from build123d import *

# Parameters (mm, degrees)
SKETCH1_W           = 104.5
SKETCH1_H           = 70
BOSS_EXTRUDE1_DEPTH = 70
SKETCH2_W           = 94.7
SKETCH2_H           = 60.2
CUT_EXTRUDE1_DEPTH  = 11
CUT_EXTRUDE3_DEPTH  = 55
SKETCH5_W           = 20
SKETCH5_H           = 10
CUT_EXTRUDE4_DEPTH  = 10


with BuildPart() as part:
    # Sketch1 → Boss-Extrude1 (new body)
    with BuildSketch(Plane(origin=(0, 0, 0), x_dir=(1, 0, 0), z_dir=(0, 1, 0))):
        with Locations((52.25, 35)):
            Rectangle(SKETCH1_W, SKETCH1_H)
    extrude(amount=BOSS_EXTRUDE1_DEPTH)

    # Sketch2 → Cut-Extrude1 (cut)
    with BuildSketch(Plane(origin=(0, 70, 0), x_dir=(1, 0, 0), z_dir=(0, 1, 0))):
        with Locations((52.2, 35)):
            Rectangle(SKETCH2_W, SKETCH2_H)
    extrude(amount=-CUT_EXTRUDE1_DEPTH, mode=Mode.SUBTRACT)

    # Sketch3 → Cut-Extrude3 (cut)
    with BuildSketch(Plane(origin=(0, 59, 0), x_dir=(1, 0, 0), z_dir=(0, 1, 0))):
        with BuildLine():
            Line((99.5, 39.153311931), (99.5, 58))
            Line((99.5, 58), (90.5, 58))
            Line((90.5, 58), (90.5, 65))
            Line((90.5, 65), (60, 65))
            Line((60, 65), (60, 58))
            Line((60, 58), (13, 58))
            Line((13, 58), (13, 65))
            Line((13, 65), (5, 65))
            Line((5, 65), (5, 57))
            Line((5, 57), (12, 57))
            Line((12, 57), (12, 12))
            Line((12, 12), (30.952452159, 12))
            ThreePointArc((30.952452159, 12), (33.5, 6.1), (36.047547841, 12))
            Line((36.047547841, 12), (65.092654993, 12))
            ThreePointArc((65.092654993, 12), (68.5, 7.7), (71.907345007, 12))
            Line((71.907345007, 12), (76.805924131, 12))
            ThreePointArc((76.805924131, 12), (82.5, 5.45), (88.194075869, 12))
            Line((88.194075869, 12), (99.5, 12))
            Line((99.5, 12), (99.5, 30.846688069))
            ThreePointArc((99.5, 30.846688069), (100, 35), (99.5, 39.153311931))
        make_face()
    extrude(amount=-CUT_EXTRUDE3_DEPTH, mode=Mode.SUBTRACT)

    # Sketch5 → Cut-Extrude4 (cut)
    with BuildSketch(Plane(origin=(104.5, 0, 0), x_dir=(0, 0, -1), z_dir=(1, 0, 0))):
        with Locations((35, 10)):
            Rectangle(SKETCH5_W, SKETCH5_H)
    extrude(amount=-CUT_EXTRUDE4_DEPTH, mode=Mode.SUBTRACT)


solid = part.part
CAD build for the part. Positions are in the model's coordinates, mm. A direction names the side the tool comes from. Coordinates: 2 decimals unless noted, no trailing zeros. Order: outer loops, then holes, each group sorted by start corner. A loop starts at its lowest first (then second) coordinate and runs counter-clockwise, first axis right, second up.
Item 1: Two-plate mould, pull along Y, no slides. Class faces 1 (the face through (52, 65, -4.9)), 2 (the face through (41, 59, -11)), 3 (the face through (102, 10, -25)): +Y half, -Y half, draft (parallel to the pull), parting line (faces both ways), or undercut.
Check sheet entries:
face 1: draft
face 2: +Y half
face 3: undercut
Item 2: Drill centre lines: L1, parallel to Z at x = 33.5, y = 25; L2, parallel to Z at x = 20, y = 31.5; L3, parallel to X at y = 26.5, z = -28.5. Where is each one in solid material? Low to high.
Check sheet entries:
L1: z = -70 to -58, -6.1 to 0
L2: z = -70 to -58, -12 to 0
L3: x = 0 to 12, 99.5 to 104.5
Item 3: Band-saw the part on B-B on x = 17. List the corners of the cut face in (y, z).
Check sheet entries:
outline: (0, -70) - (70, -70) - (70, -65.1) - (59, -65.1) - (59, -58) - (4, -58) - (4, -12) - (59, -12) - (59, -4.9) - (70, -4.9) - (70, 0) - (0, 0) - close
Item 4: Band-saw the part on D-D on y = 63.5. List the corners of the cut face in (x, z).
Check sheet entries:
outline: (0, -70) - (104.5, -70) - (104.5, 0) - (0, 0) - close; hole (4.85, -65.1) - (99.55, -65.1) - (99.55, -4.9) - (4.85, -4.9) - close
Item 5: Band-saw the part on C-C on z = -22. List the corners of the cut face in (x, y), plus the area to 3 significant figures.
Check sheet entries:
outline: (0, 0) - (104.5, 0) - (104.5, 70) - (99.55, 70) - (99.55, 59) - (99.5, 59) - (99.5, 4) - (12, 4) - (12, 59) - (4.85, 59) - (4.85, 70) - (0, 70) - close
area: 1,460 mm2
Item 6: Band-saw the part on A-A on y = 29. List the corners of the cut face in (x, z), plus the area to 3 significant figures.
Check sheet entries:
outline: (0, -70) - (104.5, -70) - (104.5, 0) - (0, 0) - close; hole (5, -65) - (13, -65) - (13, -58) - (60, -58) - (60, -65) - (90.5, -65) - (90.5, -58) - (99.5, -58) - (99.5, -39.15) arc R17.5 ccw to (99.5, -30.85) - (99.5, -12) - (88.19, -12) arc R5.75 ccw (long way) to (76.81, -12) - (71.91, -12) arc R3.5 ccw (long way) to (65.09, -12) - (36.05, -12) arc R3.5 ccw (long way) to (30.95, -12) - (12, -12) - (12, -57) - (5, -57) - close
area: 2,890 mm2
Item 7: 3-axis set-ups, long thin cutter, end or side, ignore diameter. For faces 4 (the face through (48, 70, -4)), 5 (the face through (90.5, 32, -61)), 6 (the face through (100, 37, -35)), 7 (the face through (102, 10, -45)), 8 (the face through (52, 35, 0)): which of +Z, -Z, +X, -X, +Y, -Y reach the whole face in a straight line?
Check sheet entries:
face 4: +Z, -Z, +X, -X, +Y
face 5: +Y
face 6: none
face 7: +X
face 8: +Z, +X, -X, +Y, -Y
Item 8: Pin check, flat tips, straight feed: pin 1 Ø3 at (y, z) = (8.5, -34.5) entering from +X; pin 2 Ø18 at (x, z) = (43.5, -32.5) entering from +Y. Stop position of each tip, or through.
Check sheet entries:
pin 1: stops at x = 12
pin 2: stops at y = 4
